Input: part model. Units: mm. Frame: model coordinates. A direction names the side the tool comes from. Give positions to 0.01 mm unless a question says otherwise; leave off trailing zeros. Loops run counter-clockwise (first coordinate to the right, second up) from the corner with the lowest first, then second, coordinate; pieces in that order, holes last.
from build123d import *

# Parameters (mm, degrees)
SKETCH1_W           = 45.5
SKETCH1_H           = 30.75
BOSS_EXTRUDE1_DEPTH = 1.5
CUT_EXTRUDE1_DEPTH  = 55.936895617
SKETCH3_W           = 10
SKETCH3_H           = 10
SKETCH3_W_2         = 8
SKETCH3_H_2         = 8
BOSS_EXTRUDE2_DEPTH = 3.25
SKETCH4_R           = 1.15
SKETCH4_R_2         = 1.2
CUT_EXTRUDE2_DEPTH  = 56.01249858


with BuildPart() as part:
    # Sketch1 → Boss-Extrude1 (new body)
    with BuildSketch(Plane(origin=(0, 0, 0), x_dir=(1, 0, 0), z_dir=(0, 1, 0))):
        with Locations((22.75, 15.375)):
            Rectangle(SKETCH1_W, SKETCH1_H)
    extrude(amount=BOSS_EXTRUDE1_DEPTH)

    # Sketch2 → Cut-Extrude1 (cut, through all)
    with BuildSketch(Plane(origin=(0, 1.5, 0), x_dir=(1, 0, 0), z_dir=(0, 1, 0))):
        Polygon((0, 0), (10, 0), (10, 22.75), (10, 30.75), (0, 30.75), align=None)
        Polygon((14, 3), (30.5, 3), (30.5, 12), (20.5, 12), (20.5, 22.75), (14, 22.75), align=None)
    extrude(amount=-CUT_EXTRUDE1_DEPTH, mode=Mode.SUBTRACT)

    # Sketch3 → Boss-Extrude2 (add)
    with BuildSketch(Plane(origin=(0, 1.5, 0), x_dir=(1, 0, 0), z_dir=(0, 1, 0))):
        with Locations((40.5, 5)):
            Rectangle(SKETCH3_W, SKETCH3_H)
        with Locations((16, 26.75)):
            Rectangle(SKETCH3_W_2, SKETCH3_H_2)
    extrude(amount=-BOSS_EXTRUDE2_DEPTH)

    # Sketch4 → Cut-Extrude2 (cut, through all)
    with BuildSketch(Plane(origin=(0, -1.75, 0), x_dir=(-1, 0, 0), z_dir=(0, -1, 0))):
        with Locations(Location((-42.25, 6.5, 0), (0, 0, 90))):
            Circle(SKETCH4_R)
        with Locations(Location((-15.79, 25, 0), (0, 0, 90))):
            Circle(SKETCH4_R_2)
    extrude(amount=-CUT_EXTRUDE2_DEPTH, mode=Mode.SUBTRACT)


solid = part.part
(1) Mould query, pull axis X, two halves, no side actions, for faces 1 (the flat face through (28, 0, -16)), 2 (the flat face through (22, 1, -3)), 3 (the flat face through (14, 1, -13)), 4 (the flat face through (12, -1, -27)). Classes: +X half, -X half, draft (parallel to the pull), parting line (faces both ways), or undercut.
Values follow:
face 1: draft
face 2: undercut
face 3: undercut
face 4: -X half
(2) Pin query (flat end, axial travel): pin 1 Ø1.4 at (x, z) = (15.79, -25) entering from -Y; pin 2 Ø1.9 at (y, z) = (-1, -26.5) entering from +X; pin 3 Ø1.4 at (y, z) = (-1, -5.5) entering from -X; pin 4 Ø6 at (x, z) = (31.5, -22) entering from -Y. Return the tip coordinate at first contact, or that it passes through.
Values follow:
pin 1: passes through
pin 2: stops at x = 20
pin 3: stops at x = 35.5
pin 4: stops at y = 0
(3) Ray query, probe 1 along X at (y, z) = (1.1, -6.5); probe 2 along Z at (x, y) = (28.5, 0.85); probe 3 along X at (y, z) = (0.4, -8). Return the intervals inside material, ascending.
Values follow:
probe 1: x = 10 to 14, 30.5 to 41.1, 43.4 to 45.5
probe 2: z = -30.75 to -12, -3 to 0
probe 3: x = 10 to 14, 30.5 to 45.5
(4) Reachability of faces 5 (the flat face through (30.5, 1, -7)), 6 (the flat face through (40, -1, -10)), 7 (the flat face through (16, 0, -22.75)) from +Z, -Z, +X, -X, +Y, -Y: full face, straight path, thin tool, end or side. Return the list, or none.
Values follow:
face 5: +Y, -Y
face 6: -Z, +X, -X, -Y
face 7: -Y
(5) Cut plane C-C (x = 42.25). Return the cut outline in (y, z), and give its area (4 significant figures).
Values follow:
outline: (-1.75, -10) - (0, -10) - (0, -30.75) - (1.5, -30.75) - (1.5, -7.65) - (-1.75, -7.65) - close; (-1.75, -5.35) - (1.5, -5.35) - (1.5, 0) - (-1.75, 0) - close
area: 56.15 mm2
(6) Cut plane D-D (y = 0.85). Return the cut outline in (x, z).
Values follow:
outline: (10, -30.75) - (45.5, -30.75) - (45.5, 0) - (10, 0) - close; hole (14, -22.75) - (20.5, -22.75) - (20.5, -12) - (30.5, -12) - (30.5, -3) - (14, -3) - close; hole circle Ø2.4 at (15.79, -25); hole circle Ø2.3 at (42.25, -6.5)
(7) Cut plane A-A (y = -1.25). Return the cut outline in (x, z).
Values follow:
outline: (12, -30.75) - (20, -30.75) - (20, -22.75) - (12, -22.75) - close; (35.5, -10) - (45.5, -10) - (45.5, 0) - (35.5, 0) - close; hole circle Ø2.4 at (15.79, -25); hole circle Ø2.3 at (42.25, -6.5)
(8) Cut plane B-B (z = -8.5). Return the cut outline in (x, y).
Values follow:
outline: (10, 0) - (14, 0) - (14, 1.5) - (10, 1.5) - close; (30.5, 0) - (35.5, 0) - (35.5, -1.75) - (45.5, -1.75) - (45.5, 1.5) - (30.5, 1.5) - close
